Verification items for the finished model (mm, model axes). A direction names the side the tool comes from. Give positions to 0.01 mm unless a question says otherwise; leave off trailing zeros. Loops run counter-clockwise (first coordinate to the right, second up) from the corner with the lowest first, then second, coordinate; pieces in that order, holes last. Notation, with made-up numbers: M 72.5,-39.75 L 127.5,-39.75 A13 ccw 127.5,-20.75 Z; hole C 9.25,6 d10. An arc over 180 degrees is marked long. Answer in a Markdown table with one row per item.
```python
from build123d import *

# Parameters (mm, degrees)
SKETCH1_W             = 220.35
SKETCH1_H             = 44
BOSS_EXTRUDE1_DEPTH   = 4.35
SKETCH2_W             = 6.35
SKETCH2_H             = 44
BOSS_EXTRUDE2_DEPTH   = 2
M4X0_7_TAPPED_HOLE2_D = 3.3


with BuildPart() as part:
    # Sketch1 → Boss-Extrude1 (new body)
    with BuildSketch(Plane(origin=(0, 0, 0), x_dir=(1, 0, 0), z_dir=(0, 1, 0))):
        with Locations((110.175, 22)):
            Rectangle(SKETCH1_W, SKETCH1_H)
    extrude(amount=BOSS_EXTRUDE1_DEPTH)

    # Sketch2 → Boss-Extrude2 (add)
    with BuildSketch(Plane(origin=(0, 4.35, 0), x_dir=(1, 0, 0), z_dir=(0, 1, 0))):
        with Locations((3.175, 22)):
            Rectangle(SKETCH2_W, SKETCH2_H)
    extrude(amount=BOSS_EXTRUDE2_DEPTH)

    # M4x0.7 Tapped Hole2 (through all)
    with Locations(Plane(origin=(0, 4.35, 0), x_dir=(1, 0, 0), z_dir=(0, 1, 0))):
        with Locations((135.35, 22), (175.35, 22)):
            Hole(M4X0_7_TAPPED_HOLE2_D / 2)


solid = part.part
```
Item 1: Tool access check on faces 1 (the flat face through (112, 4.35, -22)), 2 (the flat face through (109, 2, -44)). Record the directions out of +Z, -Z, +X, -X, +Y, -Y that give a thin tool (end or side, any length) a straight path to the whole face; none if there is none.
Reported:
| item | result |
|---|---|
| face 1 | +Z, -Z, +X, +Y |
| face 2 | -Z, +X, -X, +Y, -Y |
Item 2: Go/stop test with flat-tipped pins: pin 1 (4 mm diameter, centred on x = 159, z = -13.5, fed in from +Y); pin 2 (0.6 mm diameter, centred on y = 5, z = -28.5, fed in from +X). Record where each tip stops, or that it passes through.
Reported:
| item | result |
|---|---|
| pin 1 | stops at y = 4.35 |
| pin 2 | stops at x = 6.35 |
Item 3: Sectioned sample at B-B (x = 149.5). Record the cut outline in (y, z), and give its area (3 significant figures).
Reported:
| item | result |
|---|---|
| outline | M 0,-44 L 4.35,-44 L 4.35,0 L 0,0 Z |
| area | 191 mm^2 |
Item 4: Scan lines: L1, parallel to X at y = 2.5, z = -22; L2, parallel to Z at x = 175.35, y = 1.65; L3, parallel to Y at x = 72, z = -13. Record each from-to range of solid material in increasing order. Write a range as [from, to].
Reported:
| item | result |
|---|---|
| L1 | x = [0, 133.7], [137, 173.7], [177, 220.35] |
| L2 | z = [-44, -23.65], [-20.35, 0] |
| L3 | y = [0, 4.35] |
Item 5: Sectioned sample at A-A (z = -38). Record the cut outline in (x, y), and give its area (3 significant figures).
Reported:
| item | result |
|---|---|
| outline | M 0,0 L 220.35,0 L 220.35,4.35 L 6.35,4.35 L 6.35,6.35 L 0,6.35 Z |
| area | 971 mm^2 |
